Geometry check sheet. Reference: the model listing, model coordinates, mm. A direction names the side the tool comes from. Round coordinates to 2 decimals unless told otherwise and drop trailing zeros. Write each loop counter-clockwise with the first axis right and the second up, starting at its lowest first coordinate (ties: lowest second). Pieces come first, ordered by that corner, then holes. Notation, with made-up numbers: M -14.5,-14 L 17.5,-14 A18 ccw 17.5,17 Z; hole C -28.5,73.25 d5. An arc over 180 degrees is marked long. Use a Markdown table: item, result.
```python
from build123d import *

# Parameters (mm, degrees)
F0_W     = 100
F0_H     = 100
F1_DEPTH = 30
F3_DEPTH = 18
F4_R     = 10
F4_R_2   = 4
F5_DEPTH = 30.001


with BuildPart() as f1:
    # F0 (on Front) → F1 (new body)
    with BuildSketch(Plane.XZ):
        with Locations((0, -50)):
            Rectangle(F0_W, F0_H)
    extrude(amount=F1_DEPTH)

    # F2 (on face) → F3 (join)
    with BuildSketch(Plane(origin=(0, 0, 0), x_dir=(-1, 0, 0), z_dir=(0, 1, 0))):
        with BuildLine():
            ThreePointArc((-35, -70), (-30.606602, -80.606602), (-20, -85))
            Line((-20, -85), (20, -85))
            ThreePointArc((20, -85), (30.606602, -80.606602), (35, -70))
            Line((35, -70), (35, -30))
            ThreePointArc((35, -30), (30.606602, -19.393398), (20, -15))
            Line((20, -15), (-20, -15))
            ThreePointArc((-20, -15), (-30.606602, -19.393398), (-35, -30))
            Line((-35, -30), (-35, -70))
        make_face()
        with BuildLine():
            Line((20, -80), (-20, -80))
            ThreePointArc((-20, -80), (-27.071068, -77.071068), (-30, -70))
            Line((-30, -70), (-30, -30))
            ThreePointArc((-30, -30), (-27.071068, -22.928932), (-20, -20))
            Line((-20, -20), (20, -20))
            ThreePointArc((20, -20), (27.071068, -22.928932), (30, -30))
            Line((30, -30), (30, -70))
            ThreePointArc((30, -70), (27.071068, -77.071068), (20, -80))
        make_face(mode=Mode.SUBTRACT)
    extrude(amount=F3_DEPTH)

    # F4 (on face) → F5 (cut, through all)
    with BuildSketch(Plane(origin=(0, 0, 0), x_dir=(-1, 0, 0), z_dir=(0, 1, 0))):
        with Locations((0, -50)):
            Circle(F4_R)
        with Locations((41.16613, -90)):
            Circle(F4_R_2)
        with Locations((41.16613, -10)):
            Circle(F4_R_2)
        with Locations((-43.004811, -90)):
            Circle(F4_R_2)
        with Locations((-43.004811, -10)):
            Circle(F4_R_2)
    extrude(amount=-F5_DEPTH, mode=Mode.SUBTRACT)


solid = f1.part
```
Item 1: Cross-section at B-B, the plane x = 6. Record the cut outline in (y, z).
Outcome:
| item | result |
|---|---|
| outline | M -30,-100 L 0,-100 L 0,-85 L 18,-85 L 18,-80 L 0,-80 L 0,-58 L -30,-58 Z; M -30,-42 L 0,-42 L 0,-20 L 18,-20 L 18,-15 L 0,-15 L 0,0 L -30,0 Z |
Item 2: Access from +Z, -Z, +X, -X, +Y, -Y to the whole of each face (thin tool, end or side, straight path). Record for faces 5 (the face through (27.15, 8.87, -23.01)), 6 (the face through (30.72, 8.87, -80.49)), 7 (the face through (-30.72, 8.87, -19.51)), 8 (the face through (0, 9, -85)).
Outcome:
| item | result |
|---|---|
| face 5 | +Y |
| face 6 | -Z, +X, +Y |
| face 7 | +Z, -X, +Y |
| face 8 | -Z, +X, -X, +Y |
Item 3: Cross-section at C-C, the plane z = -90. Record the cut outline in (x, y), and give its area (3 significant figures).
Outcome:
| item | result |
|---|---|
| outline | M -50,-30 L -45.17,-30 L -45.17,0 L -50,0 Z; M -37.17,-30 L 39,-30 L 39,0 L -37.17,0 Z; M 47,-30 L 50,-30 L 50,0 L 47,0 Z |
| area | 2,520 mm2 |
Item 4: Mould release check, pull along X, two halves, no side actions. Record for faces 1 (the face through (-30, 9, -50)), 2 (the face through (30.49, 8.87, -19.28)), 3 (the face through (-31, 18, -47)), 4 (the face through (-35, 9, -50)): +X half, -X half, draft (parallel to the pull), parting line (faces both ways), or undercut.
Outcome:
| item | result |
|---|---|
| face 1 | undercut |
| face 2 | +X half |
| face 3 | draft |
| face 4 | -X half |
Item 5: Material ranges on line 1 along Z through (x, y) = (0, -22.5); line 2 along Z through (x, y) = (6, 10.5); line 3 along Y through (x, z) = (-43, -69.5), recorded low to high. Write a range as from..to.
Outcome:
| item | result |
|---|---|
| line 1 | z = -100..-60, -40..0 |
| line 2 | z = -85..-80, -20..-15 |
| line 3 | y = -30..0 |
Item 6: Cross-section at A-A, the plane y = -21.5. Record the cut outline in (x, z).
Outcome:
| item | result |
|---|---|
| outline | M -50,-100 L 50,-100 L 50,0 L -50,0 Z; hole C -41.17,-90 d8; hole C -41.17,-10 d8; hole C 0,-50 d20; hole C 43,-90 d8; hole C 43,-10 d8 |
Item 7: Go/stop test with flat-tipped pins: pin 1 (10.5 mm diameter, centred on x = 43, z = -10, fed in from +Y); pin 2 (6.5 mm diameter, centred on x = -41.17, z = -90, fed in from -Y); pin 3 (5.5 mm diameter, centred on y = 11.5, z = -47, fed in from -X); pin 4 (14.5 mm diameter, centred on x = -5, y = 10, fed in from -Z). Record where each tip stops, or that it passes through.
Outcome:
| item | result |
|---|---|
| pin 1 | stops at y = 0 |
| pin 2 | passes through |
| pin 3 | stops at x = -35 |
| pin 4 | stops at z = -85 |
Item 8: Cross-section at D-D, the plane z = -55.5. Record the cut outline in (x, y), and give its area (3 significant figures).
Outcome:
| item | result |
|---|---|
| outline | M -50,-30 L -8.35,-30 L -8.35,0 L -30,0 L -30,18 L -35,18 L -35,0 L -50,0 Z; M 8.35,-30 L 50,-30 L 50,0 L 35,0 L 35,18 L 30,18 L 30,0 L 8.35,0 Z |
| area | 2,680 mm2 |
